from build123d import *

# Parameters (mm, degrees)
CROQUIS1_R              = 1.5
SALIENTE_EXTRUIR1_DEPTH = 12
CROQUIS2_R              = 1.5
CORTAR_EXTRUIR1_DEPTH   = 26.442992774


with BuildPart() as part:
    # Croquis1 → Saliente-Extruir1 (new body)
    with BuildSketch(Plane.XY):
        with BuildLine():
            ThreePointArc((-14.13022151, -7.505787105), (-11.775764132, -7.307322196), (-9.712736286, -6.155465444))
            ThreePointArc((-9.712736286, -6.155465444), (-8.990280217, -7.169509232), (-8.162422223, -8.09949779))
            ThreePointArc((-8.162422223, -8.09949779), (-9.744466405, -9.854488979), (-10.461871439, -12.105752599))
            ThreePointArc((-10.461871439, -12.105752599), (-9.97583683, -12.509303719), (-9.474250703, -12.893353854))
            ThreePointArc((-9.474250703, -12.893353854), (-7.439068601, -11.692982379), (-6.080116654, -9.760081069))
            ThreePointArc((-6.080116654, -9.760081069), (-4.989229116, -10.360241012), (-3.839847924, -10.838937629))
            ThreePointArc((-3.839847924, -10.838937629), (-4.50375834, -13.106553299), (-4.173331264, -15.446142112))
            ThreePointArc((-4.173331264, -15.446142112), (-3.560334943, -15.598846595), (-2.94178835, -15.727233746))
            ThreePointArc((-2.94178835, -15.727233746), (-1.6289743, -13.762703997), (-1.24325535, -11.43159294))
            ThreePointArc((-1.24325535, -11.43159294), (0, -11.499), (1.24325535, -11.43159294))
            ThreePointArc((1.24325535, -11.43159294), (1.6289743, -13.762703997), (2.94178835, -15.727233746))
            ThreePointArc((2.94178835, -15.727233746), (3.560334943, -15.598846595), (4.173331264, -15.446142112))
            ThreePointArc((4.173331264, -15.446142112), (4.50375834, -13.106553299), (3.839847924, -10.838937629))
            ThreePointArc((3.839847924, -10.838937629), (4.989229116, -10.360241012), (6.080116654, -9.760081069))
            ThreePointArc((6.080116654, -9.760081069), (7.439068601, -11.692982379), (9.474250703, -12.893353854))
            ThreePointArc((9.474250703, -12.893353854), (9.97583683, -12.509303719), (10.461871439, -12.105752599))
            ThreePointArc((10.461871439, -12.105752599), (9.744466405, -9.854488979), (8.162422223, -8.09949779))
            ThreePointArc((8.162422223, -8.09949779), (8.990280217, -7.169509232), (9.712736286, -6.155465444))
            ThreePointArc((9.712736286, -6.155465444), (11.775764132, -7.307322196), (14.13022151, -7.505787105))
            ThreePointArc((14.13022151, -7.505787105), (14.415501886, -6.942139826), (14.678309669, -6.367670316))
            ThreePointArc((14.678309669, -6.367670316), (13.055163391, -4.65062226), (10.868328696, -3.75585308))
            ThreePointArc((10.868328696, -3.75585308), (11.210696062, -2.55876822), (11.421629379, -1.331684395))
            ThreePointArc((11.421629379, -1.331684395), (13.780125156, -1.474357234), (15.987528652, -0.631607167))
            ThreePointArc((15.987528652, -0.631607167), (16, 0), (15.987528652, 0.631607167))
            ThreePointArc((15.987528652, 0.631607167), (13.780125156, 1.474357234), (11.421629379, 1.331684395))
            ThreePointArc((11.421629379, 1.331684395), (11.210696062, 2.55876822), (10.868328696, 3.75585308))
            ThreePointArc((10.868328696, 3.75585308), (13.055163391, 4.65062226), (14.678309669, 6.367670316))
            ThreePointArc((14.678309669, 6.367670316), (14.415501886, 6.942139826), (14.13022151, 7.505787105))
            ThreePointArc((14.13022151, 7.505787105), (11.775764132, 7.307322196), (9.712736286, 6.155465444))
            ThreePointArc((9.712736286, 6.155465444), (8.990280217, 7.169509232), (8.162422223, 8.09949779))
            ThreePointArc((8.162422223, 8.09949779), (9.744466405, 9.854488979), (10.461871439, 12.105752599))
            ThreePointArc((10.461871439, 12.105752599), (9.97583683, 12.509303719), (9.474250703, 12.893353854))
            ThreePointArc((9.474250703, 12.893353854), (7.439068601, 11.692982379), (6.080116654, 9.760081069))
            ThreePointArc((6.080116654, 9.760081069), (4.989229116, 10.360241012), (3.839847924, 10.838937629))
            ThreePointArc((3.839847924, 10.838937629), (4.50375834, 13.106553299), (4.173331264, 15.446142112))
            ThreePointArc((4.173331264, 15.446142112), (3.560334943, 15.598846595), (2.94178835, 15.727233746))
            ThreePointArc((2.94178835, 15.727233746), (1.6289743, 13.762703997), (1.24325535, 11.43159294))
            ThreePointArc((1.24325535, 11.43159294), (0, 11.499), (-1.24325535, 11.43159294))
            ThreePointArc((-1.24325535, 11.43159294), (-1.6289743, 13.762703997), (-2.94178835, 15.727233746))
            ThreePointArc((-2.94178835, 15.727233746), (-3.560334943, 15.598846595), (-4.173331264, 15.446142112))
            ThreePointArc((-4.173331264, 15.446142112), (-4.50375834, 13.106553299), (-3.839847924, 10.838937629))
            ThreePointArc((-3.839847924, 10.838937629), (-4.989229116, 10.360241012), (-6.080116654, 9.760081069))
            ThreePointArc((-6.080116654, 9.760081069), (-7.439068601, 11.692982379), (-9.474250703, 12.893353854))
            ThreePointArc((-9.474250703, 12.893353854), (-9.97583683, 12.509303719), (-10.461871439, 12.105752599))
            ThreePointArc((-10.461871439, 12.105752599), (-9.744466405, 9.854488979), (-8.162422223, 8.09949779))
            ThreePointArc((-8.162422223, 8.09949779), (-8.990280217, 7.169509232), (-9.712736286, 6.155465444))
            ThreePointArc((-9.712736286, 6.155465444), (-11.775764132, 7.307322196), (-14.13022151, 7.505787105))
            ThreePointArc((-14.13022151, 7.505787105), (-14.415501886, 6.942139826), (-14.678309669, 6.367670316))
            ThreePointArc((-14.678309669, 6.367670316), (-13.055163391, 4.65062226), (-10.868328696, 3.75585308))
            ThreePointArc((-10.868328696, 3.75585308), (-11.210696062, 2.55876822), (-11.421629379, 1.331684395))
            ThreePointArc((-11.421629379, 1.331684395), (-13.780125156, 1.474357234), (-15.987528652, 0.631607167))
            ThreePointArc((-15.987528652, 0.631607167), (-16, 0), (-15.987528652, -0.631607167))
            ThreePointArc((-15.987528652, -0.631607167), (-13.780125156, -1.474357234), (-11.421629379, -1.331684395))
            ThreePointArc((-11.421629379, -1.331684395), (-11.210696062, -2.55876822), (-10.868328696, -3.75585308))
            ThreePointArc((-10.868328696, -3.75585308), (-13.055163391, -4.65062226), (-14.678309669, -6.367670316))
            ThreePointArc((-14.678309669, -6.367670316), (-14.415501886, -6.942139826), (-14.13022151, -7.505787105))
        make_face()
        Circle(CROQUIS1_R, mode=Mode.SUBTRACT)
    extrude(amount=SALIENTE_EXTRUIR1_DEPTH)

    # Croquis2 → Cortar-Extruir1 (cut, through all)
    with BuildSketch(Plane(origin=(0, 0, 0), x_dir=(-1, 0, 0), z_dir=(0, 0, -1))):
        with Locations((0, 7)):
            Circle(CROQUIS2_R)
        with Locations((0, -7)):
            Circle(CROQUIS2_R)
    extrude(amount=-CORTAR_EXTRUIR1_DEPTH, mode=Mode.SUBTRACT)


solid = part.part
Here's how the part is built. I have some questions about the finished solid (model axes, mm). A direction names the side the tool comes from. Coordinates: 2 decimals unless noted, no trailing zeros. Loops run counter-clockwise (first coordinate to the right, second up) from the corner with the lowest first, then second, coordinate; pieces in that order, holes last. Notation, with made-up numbers: (84.5, -28.75) -> (115.5, -28.75) arc R5 cw to (115.5, -22.75) -> close; hole circle Ø9 at (7, 73). An arc over 180 degrees is marked (long way). Use one line per item in the form item = value. Start each with the question number.
(1) If we section it at A-A (x = 0): Please give me the cut outline in (y, z), then the cut area to 3 significant figures.
(2) If we section it at C-C (x = 12.5): Please give me the cut outline in (y, z), then the cut area to 3 significant figures.
(3) If we section it at B-B (y = 7): Please give me the cut outline in (x, z).
(4) We'd pull the mould along Y, two halves only. Please class faces 3 (the face through (-9.969, 12.515, 5.916)), 4 (the face through (-4.97, 10.37, 5.92)), 5 (the face through (14.41, -6.95, 5.92)), 6 (the face through (5.005, 10.353, 5.916)): pulls with the +Y half, pulls with the -Y half, needs draft (parallel to the pull), parting line crosses it, or undercut.
(5) If we section it at D-D (z = 5.25): Give the number of separate pieces and of enclosed holes in the cut face, then the cut area to 3 significant figures.
(6) Please list where these lines run through material, in increasing order: line 1 along X through (y, z) = (6.5, 8.75); line 2 along Y through (x, z) = (12.5, 4.75); line 3 along X through (y, z) = (-11, 2.25).
(7) Will these pins go through, and if not, where does the flat tip stop? pin 1 (1 mm diameter, centred on y = 4.5, z = 10, fed in from -X); pin 2 (4 mm diameter, centred on x = 0, z = 7.5, fed in from -Y); pin 3 (3 mm diameter, centred on x = -1, z = 1.5, fed in from +Y).
(8) On a 3-axis mill with a long thin cutter (end or side, diameter ignored), from which of +Z, -Z, +X, -X, +Y, -Y can I reach the whole of each face in a straight line? I mean faces 1 (the face through (-11.744, 7.297, 5.916)), 2 (the face through (9.969, -12.515, 5.916)). Say none if no direction works.
Verdict:
q1.outline = (-11.5, 0) -> (-8.5, 0) -> (-8.5, 12) -> (-11.5, 12) -> close; (-5.5, 0) -> (-1.5, 0) -> (-1.5, 12) -> (-5.5, 12) -> close; (1.5, 0) -> (5.5, 0) -> (5.5, 12) -> (1.5, 12) -> close; (8.5, 0) -> (11.5, 0) -> (11.5, 12) -> (8.5, 12) -> close
q1.area = 168 mm²
q2.outline = (-7.48, 0) -> (-4.32, 0) -> (-4.32, 12) -> (-7.48, 12) -> close; (-1.52, 0) -> (1.52, 0) -> (1.52, 12) -> (-1.52, 12) -> close; (4.32, 0) -> (7.48, 0) -> (7.48, 12) -> (4.32, 12) -> close
q2.area = 112 mm²
q3.outline = (-14.39, 0) -> (-10.99, 0) -> (-10.99, 12) -> (-14.39, 12) -> close; (-9.12, 0) -> (-1.5, 0) -> (-1.5, 12) -> (-9.12, 12) -> close; (1.5, 0) -> (9.12, 0) -> (9.12, 12) -> (1.5, 12) -> close; (10.99, 0) -> (14.39, 0) -> (14.39, 12) -> (10.99, 12) -> close
q4.face_3 = pulls with the +Y half
q4.face_4 = undercut
q4.face_5 = pulls with the -Y half
q4.face_6 = undercut
q5.separate_pieces = 1
q5.enclosed_holes = 3
q5.area = 561 mm²
q6.line_1 = -14.62 to -10.15, -9.49 to -1.41, 1.41 to 9.49, 10.15 to 14.62
q6.line_2 = -7.48 to -4.32, -1.52 to 1.52, 4.32 to 7.48
q6.line_3 = -10.24 to -6.8, -3.92 to 3.92, 6.8 to 10.24
q7.pin_1 = -13.51
q7.pin_2 = -14.53
q7.pin_3 = 15.25
q8.face_1 = +Z, -Z
q8.face_2 = +Z, -Z, +X, -Y
